Input: part model. Units: mm. Frame: model coordinates. Face numbers are marked on the shaded views. A direction names the side the tool comes from. Give positions to 0.01 mm unless a question says otherwise; leave off trailing zeros. Answer in a Markdown table with one row per item. Add a question column.
1. Access query for the marked faces 1, 2, 3 and 4. Directions: +Z, -Z, +X, -X, +Y, -Y. A direction counts if a zero-diameter tool reaches every point of the face in a straight line with its end or side. Return the directions, or none.
2. Contact query for flat-ended pins moving along their axis: pin 1 (8 mm diameter, centred on y = -43.5, z = 15, fed in from -X); pin 2 (1 mm diameter, centred on x = -8, y = -19.5, fed in from +Z); pin 3 (6 mm diameter, centred on x = 30, y = -58.5, fed in from +Z). Output: stop coordinate, or through.
3. Section query A-A on y = -6.5. Count the separate pieces of the cut face and the enclosed holes in it, and give its area (3 significant figures).
4. Ray query, line 1 (Z direction, x = 0, y = -9); line 2 (Z direction, x = 15, y = -40.5); line 3 (X direction, y = -45, z = -11.5). Return the intervals inside material, ascending. Write a range as [from, to].
5. Mould query, pull axis X, two halves, no side actions, for the marked faces 5, 6 and 7. Classes: released by +X, released by -X, zero draft, split by the parting line, or undercut.
```python
from build123d import *

# Parameters (mm, degrees)
F0_R            = 41.3322868319
F1_DEPTH        = 76.2
F2_W            = 25.4
F2_H            = 25.4
F3_DEPTH        = 25.4
F3_COPIES_COUNT = 16
F4_SIZE         = 5.08
F6_D            = 12.7
F7_R            = 4.7625
F8_DEPTH        = 76.2


# Not quite as in the source:
# - a pattern or mirror of a feature is missing from the dataset's text; its kind, count and spacing are read off the source's solid


with BuildPart() as f1:
    # F0 (on Front) → F1 (new body)
    with BuildSketch(Plane.XZ):
        Circle(F0_R)
    extrude(amount=F1_DEPTH)

    # F2 (on face) → F3 (cut)
    with BuildSketch(Plane.XZ.offset(76.2)):
        with Locations((38.1, 38.1)):
            Rectangle(F2_W, F2_H)
    f3 = extrude(amount=-F3_DEPTH, mode=Mode.SUBTRACT)

    # F3_copies: F3 ×16 about axis
    f3_copies_axis = Axis((0, 0, 0), (0, 1, 0))
    for i in range(1, F3_COPIES_COUNT):
        add(f3.rotate(f3_copies_axis, i * 360 / F3_COPIES_COUNT), mode=Mode.SUBTRACT)

    # F4
    f4_edges = [f1.edges().sort_by_distance(p)[0] for p in [
        (-41.332287, 0, 0),
    ]]
    chamfer(f4_edges, length=F4_SIZE)

    # F6 (through all)
    with Locations(Plane.XZ.offset(76.2)):
        with Locations((0, 0)):
            Hole(F6_D / 2)

    # F7 (on face) → F8 (cut, through all)
    with BuildSketch(Plane.XZ.offset(76.2)):
        with Locations((17.4625, -12.6960306297)):
            Circle(F7_R)
    extrude(amount=-F8_DEPTH, mode=Mode.SUBTRACT)


solid = f1.part
```
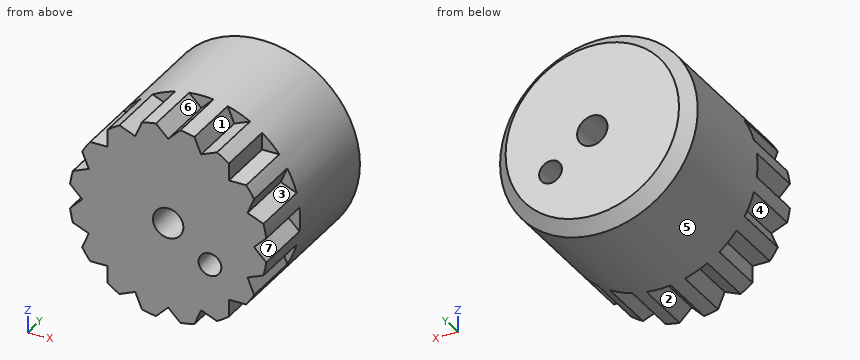
Answer:
| question | item | result |
|---|---|---|
| 1 | face 1 | +Z, -Y |
| 1 | face 2 | -Z, -Y |
| 1 | face 3 | +X, -Y |
| 1 | face 4 | -X, -Y |
| 2 | pin 1 | stops at x = -39.84 |
| 2 | pin 2 | stops at z = 40.65 |
| 2 | pin 3 | stops at z = 25.4 |
| 3 | separate pieces | 1 |
| 3 | enclosed holes | 2 |
| 3 | area | 5,170 mm² |
| 4 | line 1 | z = [-41.33, -6.35], [6.35, 41.33] |
| 4 | line 2 | z = [-38.51, -16.77], [-8.62, 38.51] |
| 4 | line 3 | x = [-39.7, 12.85], [22.07, 39.7] |
| 5 | face 5 | split by the parting line |
| 5 | face 6 | undercut |
| 5 | face 7 | released by +X |
